Check sheet for the modelled part. Datum: model origin and axes. Units: mm. Face numbers are marked on the shaded views. A direction names the side the tool comes from. Round coordinates to 2 decimals unless told otherwise and drop trailing zeros. Order: outer loops, then holes, each group sorted by start corner. A loop starts at its lowest first (then second) coordinate and runs counter-clockwise, first axis right, second up.
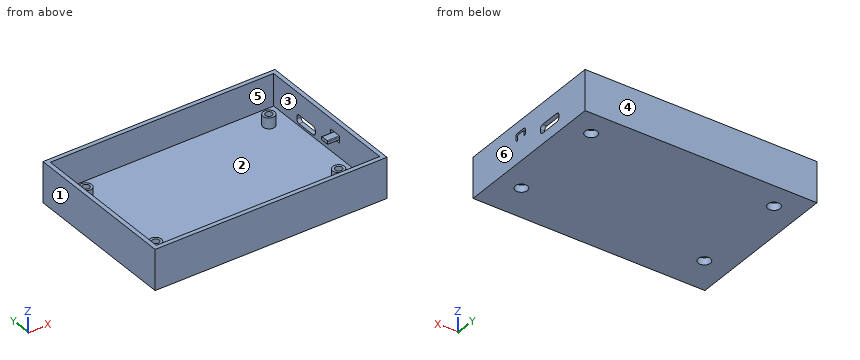
Solid Edge part; units mm, degrees
sketch "Sketch1" plane through (0, 0, 0) normal (0, 0, 1) x (1, 0, 0)
  line L0 (-54.5, -37) -> (54.5, -37)
  line L1 (54.5, -37) -> (54.5, 37)
  line L2 (54.5, 37) -> (-54.5, 37)
  line L3 (-54.5, 37) -> (-54.5, -37)
extrude "Protrusion1" add sketch "Sketch1" against normal blind 4
sketch "Sketch2" plane through (0, 0, 0) normal (0, 0, 1) x (1, 0, 0)
  line L0 (-54.5, 37) -> (-54.5, -37)
  line L1 (-54.5, -37) -> (54.5, -37)
  line L2 (54.5, -37) -> (54.5, 37)
  line L3 (54.5, 37) -> (-54.5, 37)
  line L4 (-52.5, 35) -> (-52.5, -35)
  line L5 (-52.5, -35) -> (52.5, -35)
  line L6 (52.5, -35) -> (52.5, 35)
  line L7 (52.5, 35) -> (-52.5, 35)
extrude "ExtrudedProtrusion_2" add sketch "Sketch2" along normal blind 15
sketch "Sketch3" plane through (54.5, 0, 5.5) normal (1, 0, 0) x (0, 1, 0)
  arc A0 (-2.5, 3.8) -> (-3.2, 4.5) centre (-3.2, 3.8) ccw
  line L0 (-7.8008, 4.5) -> (-3.2, 4.5)
  arc A1 (-7.8008, 4.5) -> (-8.5, 3.8008) centre (-7.8008, 3.8008) ccw
  line L1 (-8.5, 1.5) -> (-8.5, 3.8008)
  line L2 (-7.5, 3.15) -> (-7.5, 1.5)
  arc A2 (-7.5, 3.15) -> (-7.15, 3.5) centre (-7.15, 3.15) cw
  line L3 (-3.8523, 3.5) -> (-7.15, 3.5)
  arc A3 (-3.8523, 3.5) -> (-3.5, 3.1477) centre (-3.8523, 3.1477) cw
  line L4 (-3.5, 1.5) -> (-3.5, 3.1477)
  line L5 (-2.5, 1.5) -> (-2.5, 3.8)
  arc A4 (-7.5, 1.5) -> (-8.5, 1.5) centre (-8, 1.5) cw
  arc A5 (-2.5, 1.5) -> (-3.5, 1.5) centre (-3, 1.5) cw
extrude "Cutout1" cut sketch "Sketch3" against normal blind 6.7422
sketch "Sketch4" plane through (0, 0, -4) normal (0, 0, -1) x (1, 0, 0)
  circle A0 centre (-42.5, 20.5) radius 2.845
  circle A1 centre (43.5, 20.5) radius 2.845
  circle A2 centre (43.5, -25.5) radius 2.845
  circle A3 centre (-42.5, -25.5) radius 2.845
extrude "ExtrudedCutout_11" cut sketch "Sketch4" against normal blind 3.3
sketch "Sketch5" plane through (0, 0, 0) normal (0, 0, 1) x (0, 1, 0)
  circle A0 centre (25.5, -43.5) radius 2.75
  circle A1 centre (25.5, 42.5) radius 2.75
  circle A2 centre (-20.5, 42.5) radius 2.75
  circle A3 centre (-20.5, -43.5) radius 2.75
extrude "ExtrudedProtrusion_15" add sketch "Sketch5" along normal blind 5
sketch "Sketch6" plane through (0, 0, -4) normal (0, 0, -1) x (1, 0, 0)
  circle A0 centre (-42.5, -25.5) radius 1.65
  circle A1 centre (-42.5, 20.5) radius 1.65
  circle A2 centre (43.5, -25.5) radius 1.65
  circle A3 centre (43.5, 20.5) radius 1.65
extrude "ExtrudedCutout_13" cut sketch "Sketch6" against normal blind 19.0818
sketch "Sketch7" plane through (54.5, 0, 5.5) normal (1, 0, 0) x (0, 1, 0)
  line L0 (19.7, -0.5) -> (7.5, -0.5)
  line L1 (7.5, -0.5) -> (7.5, -4.5)
  line L2 (7.5, -4.5) -> (19.7, -4.5)
  line L3 (19.7, -4.5) -> (19.7, -0.5)
extrude "Cutout2" cut sketch "Sketch7" against normal up to next
fillet "Round_5" radius 1.5 4 edges at (53.5, 19.7, 5) (53.5, 19.7, 1) (53.5, 7.5, 1) (53.5, 7.5, 5)
sketch "Sketch8" plane through (52.5, 0, 7.5) normal (-1, 0, 0) x (0, -1, 0)
  line L0 (3.5, 0) -> (7.5, 0)
  line L1 (7.5, 0) -> (7.5, -0.5)
  arc A0 (7.5, -0.5) -> (8, -1) centre (8, -0.5) ccw
  line L2 (3, -1) -> (8, -1)
  arc A1 (3.5, -0.5) -> (3, -1) centre (3, -0.5) cw
  line L3 (3.5, -0.5) -> (3.5, 0)
extrude "ExtrudedCutout_15" cut sketch "Sketch8" against normal blind 1
sketch "Sketch9" plane through (52.5, -5.5, 8.25) normal (-1, 0, 0) x (0, -1, 0)
  line L0 (2, -0.75) -> (2, 0.4)
  line L1 (-2, -0.75) -> (2, -0.75)
  line L2 (-2, 0.3977) -> (-2, -0.75)
  line L3 (-1.6477, 0.75) -> (1.65, 0.75)
  arc A0 (1.65, 0.75) -> (2, 0.4) centre (1.65, 0.4) cw
  arc A1 (-2, 0.3977) -> (-1.6477, 0.75) centre (-1.6477, 0.3977) cw
extrude "ExtrudedProtrusion_16" add sketch "Sketch9" along normal blind 4.9
1) Scan lines: line 1 (X direction, y = 25.5, z = 2.4); line 2 (Y direction, x = -42.5, z = 3.3); line 3 (X direction, y = 25.5, z = -2.15) (3 decimals). Record each from-to range of solid material in increasing order.
2) Sectioned sample at B-B on y = 25.5. Count the separate pieces of the cut face and the enclosed holes in it, and give its area (3 significant figures).
3) Set-up check for the marked faces 5 and 6: record each of +Z, -Z, +X, -X, +Y, -Y from which the full face is reachable in a straight line by a thin tool's end or side.
4) Draft check along Y on the marked faces 1, 2, 3 and 4. Enter one of: pulls with the +Y half, pulls with the -Y half, needs draft (parallel to the pull), parting line crosses it, or undercut.
5) Sectioned sample at A-A on y = 12.5. Record the cut outline in (x, z).
6) Sectioned sample at C-C on x = -38.5. Record the cut outline in (y, z).
7) Gauge pin test, flat end, axial feed: pin 1 (3 mm diameter, centred on x = 43, y = -19.5, fed in from +Z). Record the tip position at first contact, or that the pin passes through.
Values found:
1. line 1: x = -54.5 to -52.5, -45.25 to -44.15, -40.85 to -39.75, 40.75 to 41.85, 45.15 to 46.25, 52.5 to 54.5
1. line 2: y = -37 to -35, -23.25 to -22.15, -18.85 to -17.75, 22.75 to 23.85, 27.15 to 28.25, 35 to 37
1. line 3: x = -54.5 to -45.345, -39.655 to 40.655, 46.345 to 54.5
2. separate pieces: 3
2. enclosed holes: 0
2. area: 476 mm2
3. face 5: +Z
3. face 6: +Z, -Z, +X, +Y, -Y
4. face 1: needs draft
4. face 2: undercut
4. face 3: undercut
4. face 4: pulls with the +Y half
5. outline: (-54.5, -4) - (54.5, -4) - (54.5, 1) - (52.5, 1) - (52.5, 0) - (-52.5, 0) - (-52.5, 15) - (-54.5, 15) - close; (52.5, 5) - (54.5, 5) - (54.5, 15) - (52.5, 15) - close
6. outline: (-37, -4) - (37, -4) - (37, 15) - (35, 15) - (35, 0) - (-35, 0) - (-35, 15) - (-37, 15) - close
7. pin 1: stops at z = 5
